Check sheet for the drawn part. Datum: minimum x, y, z corner. Units: mm. A direction names the side the tool comes from. Give positions to 0.01 mm unless a question says otherwise; leave off trailing zeros. Write each loop counter-clockwise with the first axis right and the second up, starting at its lowest first coordinate (ties: lowest second). Pieces come first, ordered by that corner, then holes. Notation, with made-up numbers: (10, 47.25) -> (40, 47.25) arc R18 ccw to (40, 68.25) -> close; hole circle Ø3 at (-39, 74). An arc over 180 degrees is marked (long way). Write item = value, one per line. Start each with the question number.
1. Cross-section at B-B, the plane y = 6.75. State how many separate pieces and enclosed holes the cut face has, plus the area to 3 significant figures.
2. Thickness scan on line 1 along X through (y, z) = (1.5, 21.5) (1 decimal); line 2 along X through (y, z) = (9.25, 14.75); line 3 along X through (y, z) = (5, 7) (1 decimal). Record the ranges inside material, lowest first.
3. Cross-section at D-D, the plane x = 16.5. Record the cut outline in (y, z), plus the area to 3 significant figures.
4. Mould release check, pull along Z, two halves, no side actions. Record for the marked faces 4, 5, 6 and 7: pulls with the +Z half, pulls with the -Z half, needs draft (parallel to the pull), parting line crosses it, or undercut.
5. Set-up check for the marked faces 1, 2 and 3: record each of +Z, -Z, +X, -X, +Y, -Y from which the full face is reachable in a straight line by a thin tool's end or side.
6. Depth check by flat-ended pin: P1, Ø5, axis at y = 7.5, z = 13, coming from the +X side; P2, Ø3, axis at y = 7.5, z = 12.5, coming from the +X side; P3, Ø1.5, axis at y = 2.5, z = 21.5, coming from the +X side; P4, Ø4, axis at x = 32.375, z = 7, coming from the +Y side. Enter the tip coordinate at first touch or a pass-through.
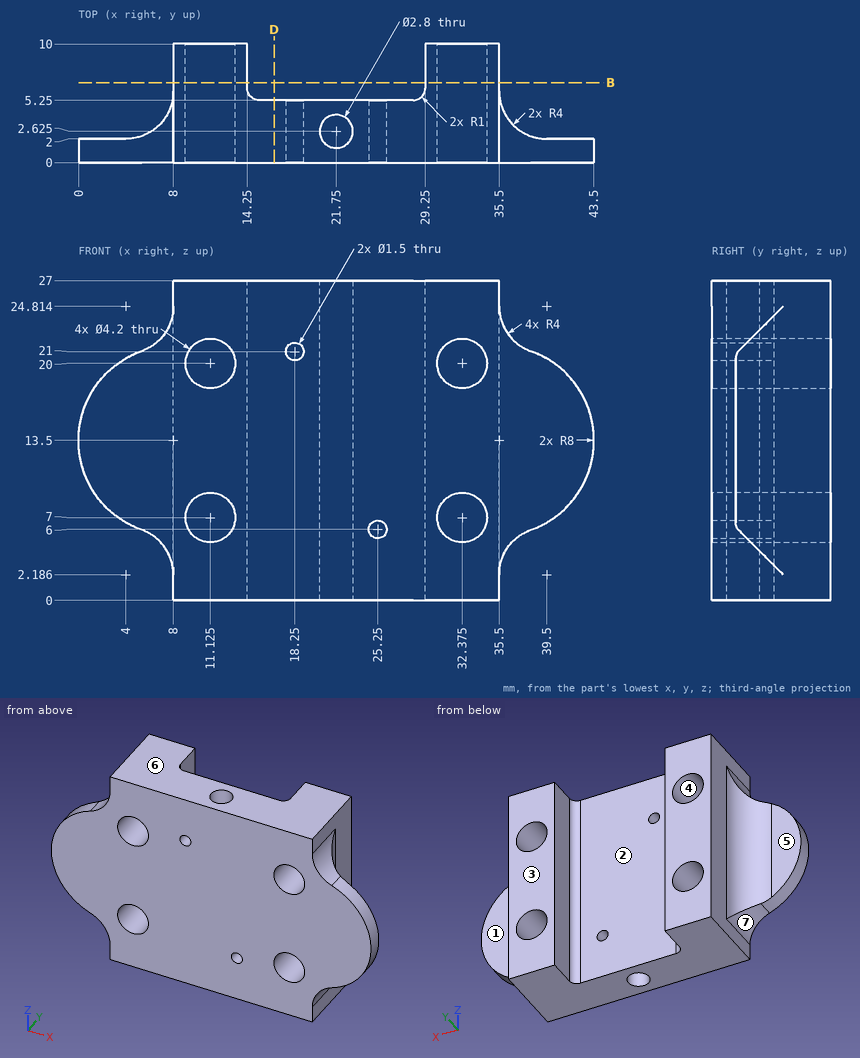
Answers:
q1.separate_pieces = 2
q1.enclosed_holes = 4
q1.area = 282 mm^2
q2.line_1 = 6.2 to 9.7, 12.6 to 17.7, 18.8 to 20.9, 22.6 to 30.9, 33.8 to 37.3
q2.line_2 = 8 to 14.25, 29.25 to 35.5
q2.line_3 = 7.9 to 9, 13.2 to 30.3, 34.5 to 35.6
q3.outline = (0, 0) -> (5.25, 0) -> (5.25, 27) -> (0, 27) -> close
q3.area = 142 mm^2
q4.face_4 = undercut
q4.face_5 = needs draft
q4.face_6 = pulls with the +Z half
q4.face_7 = pulls with the -Z half
q5.face_1 = +Z, -Z, +X, +Y
q5.face_2 = +Z, -Z, +Y
q5.face_3 = +Z, -Z, +X, -X, +Y
q6.P1 = 35.63
q6.P2 = 35.5
q6.P3 = 38.62
q6.P4 = through
